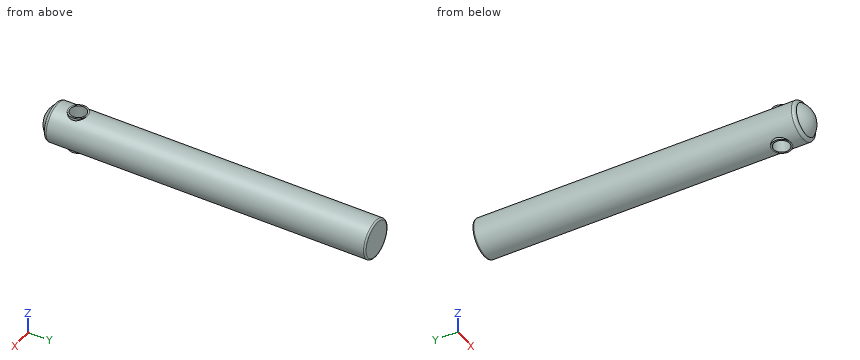
from build123d import *

# Parameters (mm, degrees)
SKETCH_1_R          = 12
EXTRUDE_1_DEPTH     = 200
EXTRUDE_START       = -24
SKETCH_2_R          = 6
EXTRUDE_2_DEPTH     = 24
CUT_EXTRUDE_1_REACH = 203.792
SKETCH_3_R          = 5
FILLET_1_R          = 2
FILLET_2_R          = 1
DOME_1_FACE_RADIUS  = 10
DOME_1_HEIGHT       = 5


with BuildPart() as part:
    # 스케치1 → 보스-돌출1 (new body)
    with BuildSketch(Plane(origin=(0, 0, 0), x_dir=(1, 0, 0), z_dir=(0, 1, 0))):
        with Locations(Location((0, 0, 0), (0, 0, 270))):
            Circle(SKETCH_1_R)
    extrude(amount=EXTRUDE_1_DEPTH)

    # 스케치2 → 보스-돌출2 (add)
    with BuildSketch(Plane.XY.offset(12).offset(EXTRUDE_START)):
        with Locations((0, 15)):
            Circle(SKETCH_2_R)
    extrude(amount=EXTRUDE_2_DEPTH)

    # 스케치3 → 컷-돌출1 (cut, up to next)
    with BuildSketch(Plane.XY.offset(12), mode=Mode.PRIVATE) as cut_extrude_1_sk1:
        with Locations((0, 15)):
            Circle(SKETCH_3_R)
    cut_extrude_1_tool1 = extrude(cut_extrude_1_sk1.sketch, amount=-CUT_EXTRUDE_1_REACH, mode=Mode.PRIVATE) & part.part
    add(cut_extrude_1_tool1.solids().sort_by_distance((0, 15, 12))[0], mode=Mode.SUBTRACT)

    # 필렛1
    fillet_1_edges = [part.edges().sort_by_distance(p)[0] for p in [
        (0, 0, -12),
    ]]
    fillet(fillet_1_edges, radius=FILLET_1_R)

    # 필렛2
    fillet_2_edges = [part.edges().sort_by_distance(p)[0] for p in [
        (0, 200, -12),
    ]]
    fillet(fillet_2_edges, radius=FILLET_2_R)

    # 돔1: a dome of height H over a round flat face of radius A is a cap of a sphere of radius (A * A + H * H) / (2 * H)
    dome_1_r = (DOME_1_FACE_RADIUS * DOME_1_FACE_RADIUS + DOME_1_HEIGHT * DOME_1_HEIGHT) / (2 * DOME_1_HEIGHT)
    dome_1_base = Plane((0, 0, 0), z_dir=(0, -1, 0))
    with Locations(dome_1_base.offset(DOME_1_HEIGHT - dome_1_r)):
        dome_1_ball = Sphere(dome_1_r, mode=Mode.PRIVATE)
    add(split(dome_1_ball, bisect_by=dome_1_base, keep=Keep.TOP, mode=Mode.PRIVATE))


solid = part.part
Design review of the part built by this model. Coordinates are the model's own, in mm. Give positions to 0.01 mm unless a question says otherwise; leave off trailing zeros. Loops run counter-clockwise (first coordinate to the right, second up) from the corner with the lowest first, then second, coordinate; pieces in that order, holes last. Notation, with made-up numbers: (-32, 74.5) -> (13, 74.5) arc R22 cw to (13, 112.5) -> close; hole circle Ø11 at (51.5, 77.5). An arc over 180 degrees is marked (long way). One line per question, with ' | ' between items. Start each with the question number.
(1) For line 1 (Y direction, x = 0, z = -1); line 2 (Z direction, x = 1, y = 123.5); line 3 (X direction, y = 175, z = 4.75), list the stretches that pass through material, from the lowest coordinate up.
(2) We need section B-B (y = 15). State the section outline as (x, z) points.
(3) Insertion check: P1, Ø8, axis at x = 8.5, y = 173.5, coming from the +Z side; P2, Ø10, axis at x = 0, z = -6, coming from the -Y side; P3, Ø4, axis at y = 29, z = 8.5, coming from the +X side. Each pin has a flat end and moves straight along its axis. Give the tip position at first contact, or say it passes through.
(4) We need section C-C (y = 126). State the section outline as (x, z) points.
(5) We need section A-A (z = 0). State the section outline as (x, y) points, and give its area (3 significant figures).
The answers:
1) line 1: y = -4.96 to 10, 20 to 200 | line 2: z = -11.96 to 11.96 | line 3: x = -11.02 to 11.02
2) outline: (-6, -12) -> (-5, -12) -> (-5, 12) -> (-6, 12) -> (-6, 10.39) arc R12 ccw to (-6, -10.39) -> close; (5, -12) -> (6, -12) -> (6, -10.39) arc R12 ccw to (6, 10.39) -> (6, 12) -> (5, 12) -> close
3) P1: stops at z = 11.12 | P2: stops at y = -4.96 | P3: stops at x = 10.09
4) outline: circle Ø24 at (0, 0)
5) outline: (-12, 2) arc R2 ccw to (-10, 0) arc R12.5 ccw to (10, 0) arc R2 ccw to (12, 2) -> (12, 199) arc R1 ccw to (11, 200) -> (-11, 200) arc R1 ccw to (-12, 199) -> close; hole circle Ø10 at (0, 15) | area: 4,790 mm^2
